Check sheet for the modelled part. Datum: model origin and axes. Units: mm. Round coordinates to 2 decimals unless told otherwise and drop trailing zeros. Order: outer loops, then holes, each group sorted by start corner. A loop starts at its lowest first (then second) coordinate and runs counter-clockwise, first axis right, second up.
(1) Sectioned sample at A-A, the plane z = 4.5. Enter the section's corners in (x, y).
(2) Sectioned sample at C-C, the plane z = 8.75. Enter the section's corners in (x, y), and give its area (3 significant figures).
(3) Depth check by flat-ended pin: pin 1 (7.5 mm diameter, centred on y = 8, z = 11, fed in from +X). Enter the tip coordinate at first touch or a pass-through.
(4) Sectioned sample at B-B, the plane y = -9.5. Enter the section's corners in (x, z), and give its area (3 significant figures).
(5) Thickness scan on probe 1 along X at (y, z) = (2.5, 14.5). Record the ranges inside material, lowest first.
```python
from build123d import *

# Parameters (mm, degrees)
F1_DEPTH = 15.2
F2_R     = 2.1
F3_DEPTH = 1.5
F4_R     = 0.2
F6_DEPTH = 0.9
F7_R     = 0.2


with BuildPart() as f1:
    # F0 (on Top) → F1 (new body)
    with BuildSketch(Plane.XY):
        with BuildLine():
            Line((19.072499, 20.445805), (-30.327501, 20.445805))
            Line((-30.327501, 20.445805), (-30.327501, -13.554195))
            Line((-30.327501, -13.554195), (19.072499, -13.554195))
            ThreePointArc((19.072499, -13.554195), (20.486712, -12.968409), (21.072499, -11.554195))
            Line((21.072499, -11.554195), (21.072499, 18.445805))
            ThreePointArc((21.072499, 18.445805), (20.486712, 19.860018), (19.072499, 20.445805))
        make_face()
    extrude(amount=F1_DEPTH)

    # F2 (on face) → F3 (join)
    with BuildSketch(Plane.YZ.offset(21.072499)):
        with Locations((3.645805, 4.5)):
            Circle(F2_R)
    extrude(amount=F3_DEPTH)

    # F4
    f4_edges = [f1.edges().sort_by_distance(p)[0] for p in [
        (21.072499, 3.445805, 15.2),
        (21.072499, 3.445805, 0),
        (22.572499, 1.545805, 4.5),
        (21.072499, 1.545805, 4.5),
        (-30.327501, 20.445805, 7.6),
        (-30.327501, -13.554195, 7.6),
        (-30.327501, 3.445805, 15.2),
        (-30.327501, 3.445805, 0),
    ]]
    fillet(f4_edges, radius=F4_R)

    # F5 (on face) → F6 (join)
    with BuildSketch(Plane.XY.offset(15.2)):
        with BuildLine():
            Line((-29.127501, 19.245805), (-29.127501, -12.354195))
            Line((-29.127501, -12.354195), (19.072499, -12.354195))
            ThreePointArc((19.072499, -12.354195), (19.638184, -12.119881), (19.872499, -11.554195))
            Line((19.872499, -11.554195), (19.872499, 18.445805))
            ThreePointArc((19.872499, 18.445805), (19.638184, 19.01149), (19.072499, 19.245805))
            Line((19.072499, 19.245805), (-29.127501, 19.245805))
        make_face()
    extrude(amount=F6_DEPTH)

    # F7
    f7_edges = [f1.edges().sort_by_distance(p)[0] for p in [
        (-5.027501, -12.354195, 16.1),
        (19.638184, -12.119881, 16.1),
        (19.872499, 3.445805, 16.1),
        (19.638184, 19.01149, 16.1),
        (-5.027501, 19.245805, 16.1),
        (-29.127501, 3.445805, 16.1),
    ]]
    fillet(f7_edges, radius=F7_R)


solid = f1.part
```
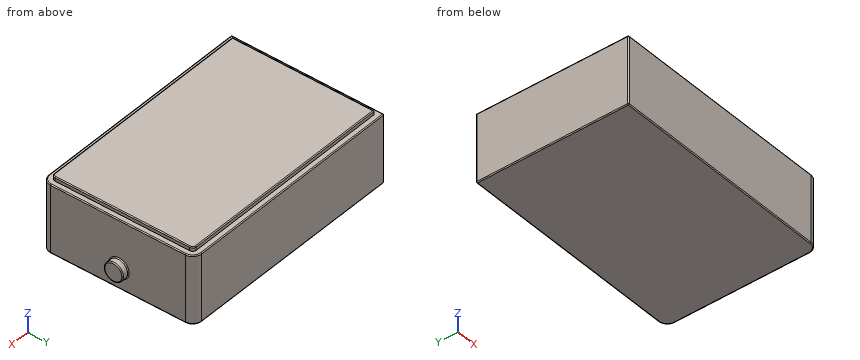
Derived:
1. outline: (-30.33, -13.35) arc R0.2 ccw to (-30.13, -13.55) - (19.07, -13.55) arc R2 ccw to (21.07, -11.55) - (21.07, 1.35) arc R0.2 cw to (21.27, 1.55) - (22.37, 1.55) arc R0.2 ccw to (22.57, 1.75) - (22.57, 5.55) arc R0.2 ccw to (22.37, 5.75) - (21.27, 5.75) arc R0.2 cw to (21.07, 5.95) - (21.07, 18.45) arc R2 ccw to (19.07, 20.45) - (-30.13, 20.45) arc R0.2 ccw to (-30.33, 20.25) - close
2. outline: (-30.33, -13.35) arc R0.2 ccw to (-30.13, -13.55) - (19.07, -13.55) arc R2 ccw to (21.07, -11.55) - (21.07, 18.45) arc R2 ccw to (19.07, 20.45) - (-30.13, 20.45) arc R0.2 ccw to (-30.33, 20.25) - close
2. area: 1,750 mm2
3. pin 1: stops at x = 21.07
4. outline: (-30.33, 0.2) arc R0.2 ccw to (-30.13, 0) - (20.87, 0) arc R0.2 ccw to (21.07, 0.2) - (21.07, 15) arc R0.2 ccw to (20.87, 15.2) - (19.87, 15.2) - (19.87, 15.9) arc R0.2 ccw to (19.67, 16.1) - (-28.93, 16.1) arc R0.2 ccw to (-29.13, 15.9) - (-29.13, 15.2) - (-30.13, 15.2) arc R0.2 ccw to (-30.33, 15) - close
4. area: 825 mm2
5. probe 1: x = -30.33 to 21.07
